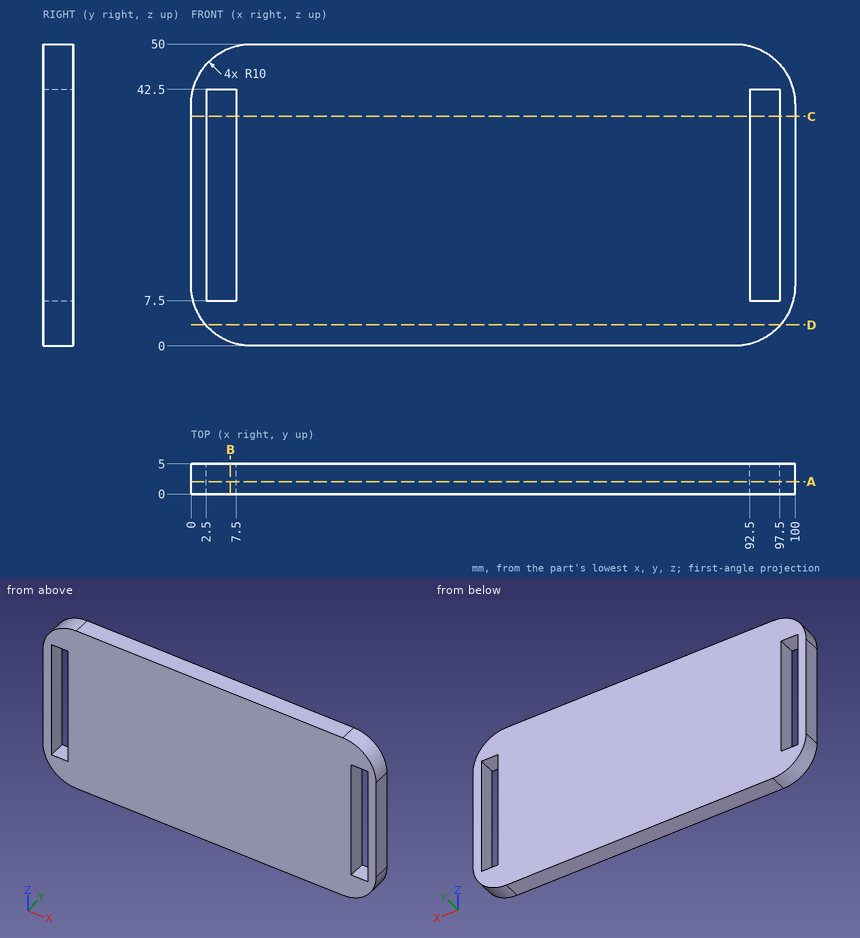
The drawing under review shows one solid part. Ordinate dimensions are in mm from its lowest x, y, z. Round coordinates to 2 decimals unless told otherwise and drop trailing zeros. Loops run counter-clockwise (first coordinate to the right, second up) from the corner with the lowest first, then second, coordinate; pieces in that order, holes last. Notation, with made-up numbers: (19.25, -9) -> (76.25, -9) arc R16 cw to (76.25, -5) -> close; hole circle Ø11 at (22, 19.5). An arc over 180 degrees is marked (long way). Answer in a Markdown table with one row per item.
1) For pin 1 Ø1 at (y, z) = (2.5, 43.5) entering from +X, flat-tipped, find the tip position at first contact; note if it passes through.
Taken from the geometry:
| item | result |
|---|---|
| pin 1 | stops at x = 99.54 |
2) Wall thickness on line 1 along X through (y, z) = (1.6, 16); line 2 along X through (y, z) = (0.55, 8); line 3 along Z through (x, y) = (4.5, 1.95): over which ranges is each line inside the solid? List them lowest first.
Taken from the geometry:
| item | result |
|---|---|
| line 1 | x = 0 to 2.5, 7.5 to 92.5, 97.5 to 100 |
| line 2 | x = 0.2 to 2.5, 7.5 to 92.5, 97.5 to 99.8 |
| line 3 | z = 1.65 to 7.5, 42.5 to 48.35 |
3) Consider section D-D, the plane z = 3.5. Write out the cut boundary in (x, y).
Taken from the geometry:
| item | result |
|---|---|
| outline | (2.4, 0) -> (97.6, 0) -> (97.6, 5) -> (2.4, 5) -> close |
4) Consider section B-B, the plane x = 6.5. Write out the cut boundary in (y, z), plus the area to 3 significant figures.
Taken from the geometry:
| item | result |
|---|---|
| outline | (0, 0.63) -> (5, 0.63) -> (5, 7.5) -> (0, 7.5) -> close; (0, 42.5) -> (5, 42.5) -> (5, 49.37) -> (0, 49.37) -> close |
| area | 68.7 mm² |
5) Consider section C-C, the plane z = 38. Write out the cut boundary in (x, y).
Taken from the geometry:
| item | result |
|---|---|
| outline | (0, 0) -> (2.5, 0) -> (2.5, 5) -> (0, 5) -> close; (7.5, 0) -> (92.5, 0) -> (92.5, 5) -> (7.5, 5) -> close; (97.5, 0) -> (100, 0) -> (100, 5) -> (97.5, 5) -> close |
6) Consider section A-A, the plane y = 2.05. Write out the cut boundary in (x, z), plus the area to 3 significant figures.
Taken from the geometry:
| item | result |
|---|---|
| outline | (0, 10) arc R10 ccw to (10, 0) -> (90, 0) arc R10 ccw to (100, 10) -> (100, 40) arc R10 ccw to (90, 50) -> (10, 50) arc R10 ccw to (0, 40) -> close; hole (2.5, 7.5) -> (7.5, 7.5) -> (7.5, 42.5) -> (2.5, 42.5) -> close; hole (92.5, 7.5) -> (97.5, 7.5) -> (97.5, 42.5) -> (92.5, 42.5) -> close |
| area | 4,560 mm² |
